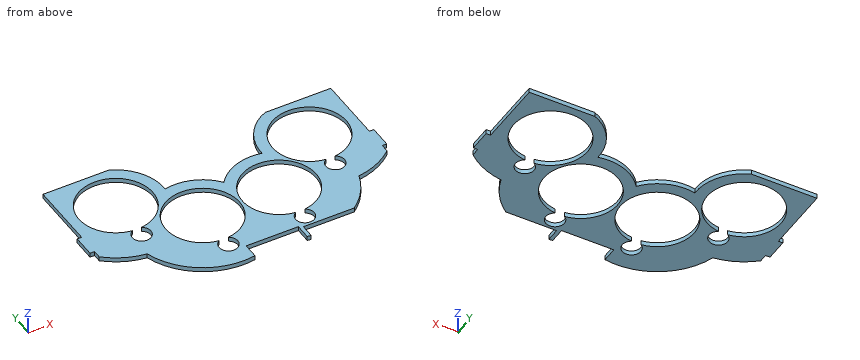
from build123d import *

# Parameters (mm, degrees)
EXTRUDE_1_DEPTH = 6


with BuildPart() as part:
    # Эскиз1 → Бобышка-Вытянуть1 (new body)
    with BuildSketch(Plane.XY):
        with BuildLine():
            Line((424, 250), (424, 160))
            Line((424, 160), (430, 160))
            Line((430, 160), (430, 130))
            Line((430, 130), (424, 130))
            Line((424, 130), (424, 118.979785419))
            ThreePointArc((424, 118.979785419), (400.249049588, 103.530628738), (372.998295097, 95.773021676))
            ThreePointArc((372.998295097, 95.773021676), (359.88843335, 69.223630945), (339.241493801, 48))
            Line((339.241493801, 48), (271, 48))
            Line((271, 48), (271, 29.720915629))
            ThreePointArc((271, 29.720915629), (268.495114821, 30.054927971), (266, 30.455447679))
            Line((266, 30.455447679), (266, 51))
            Line((266, 51), (196, 51))
            Line((196, 51), (196, 30.455447679))
            ThreePointArc((196, 30.455447679), (130.198007186, 42.960646788), (89.001704904, 95.773021676))
            ThreePointArc((89.001704904, 95.773021676), (61.750950412, 103.530628738), (38, 118.979785419))
            Line((38, 118.979785419), (38, 130))
            Line((38, 130), (32, 130))
            Line((32, 130), (32, 160))
            Line((32, 160), (38, 160))
            Line((38, 160), (38, 250))
            Line((38, 250), (126.096189432, 250))
            ThreePointArc((126.096189432, 250), (155.836604626, 225.049778093), (166.051782667, 187.59772866))
            ThreePointArc((166.051782667, 187.59772866), (201.928287817, 185.126127233), (231, 163.958510782))
            ThreePointArc((231, 163.958510782), (260.071712183, 185.126127233), (295.948217333, 187.59772866))
            ThreePointArc((295.948217333, 187.59772866), (306.163395374, 225.049778093), (335.903810568, 250))
            Line((335.903810568, 250), (424, 250))
        make_face()
        with BuildLine():
            ThreePointArc((107.24460838, 140.883333333), (101.096189432, 239.5), (94.947770485, 140.883333333))
            ThreePointArc((94.947770485, 140.883333333), (101.096189432, 117.5), (107.24460838, 140.883333333))
        make_face(mode=Mode.SUBTRACT)
        with BuildLine():
            ThreePointArc((185.845397449, 74.929440215), (179.696978501, 173.546106882), (173.548559554, 74.929440215))
            ThreePointArc((173.548559554, 74.929440215), (179.696978501, 51.546106882), (185.845397449, 74.929440215))
        make_face(mode=Mode.SUBTRACT)
        with BuildLine():
            ThreePointArc((288.451440446, 74.929440215), (282.303021499, 173.546106882), (276.154602551, 74.929440215))
            ThreePointArc((276.154602551, 74.929440215), (282.303021499, 51.546106882), (288.451440446, 74.929440215))
        make_face(mode=Mode.SUBTRACT)
        with BuildLine():
            ThreePointArc((367.052229515, 140.883333333), (360.903810568, 239.5), (354.75539162, 140.883333333))
            ThreePointArc((354.75539162, 140.883333333), (360.903810568, 117.5), (367.052229515, 140.883333333))
        make_face(mode=Mode.SUBTRACT)
    extrude(amount=EXTRUDE_1_DEPTH)


solid = part.part
Geometry: final body of the model. Coordinates: model frame, mm. Give positions to 0.01 mm unless a question says otherwise; leave off trailing zeros. Loops run counter-clockwise (first coordinate to the right, second up) from the corner with the lowest first, then second, coordinate; pieces in that order, holes last. Notation, with made-up numbers: (-35, 61) - (-6, 61) arc R20 ccw to (-6, 92) - close; hole circle Ø10 at (45.25, 86). An arc over 180 degrees is marked (long way). Answer as CSV lines item,"result". Start each with the question number.
1. Section A-A, the plane y = 178. Return loops of the section in (x, z), plus the area to 3 significant figures.
2. Ray query, L1, parallel to Y at x = 290, z = 5; L2, parallel to X at y = 211, z = 1.95; L3, parallel to X at y = 102, z = 5.7. Return the intervals inside material, ascending.
3. Section C-C, the plane x = 146.5. Return loops of the section in (y, z).
4. Pin query (flat end, axial travel): P1, Ø3, axis at y = 123.5, z = 3.5, coming from the +X side; P2, Ø3, axis at x = 36, z = 2, coming from the +Y side. Return the tip coordinate at first contact, or that it passes through.
5. Section B-B, the plane z = 3.3. Give the number of separate pieces and of enclosed holes in the cut face, plus the area to 3 significant figures.
6. Section D-D, the plane y = 100.5. Return loops of the section in (x, z), plus the area to 3 significant figures.
Answers:
1,outline,"(38, 0) - (53.07, 0) - (53.07, 6) - (38, 6) - close; (149.12, 0) - (215.95, 0) - (215.95, 6) - (149.12, 6) - close; (246.05, 0) - (312.88, 0) - (312.88, 6) - (246.05, 6) - close; (408.93, 0) - (424, 0) - (424, 6) - (408.93, 6) - close"
1,area,"983 mm2"
2,L1,"y = 48 to 54.2, 73.9 to 75.15, 172.94 to 188.59"
2,L2,"x = 38 to 56.27, 145.92 to 162.61, 299.39 to 316.08, 405.73 to 424"
2,L3,"x = 65.31 to 135.38, 224.02 to 237.98, 326.62 to 396.69"
3,outline,"(35.04, 0) - (87.33, 0) - (87.33, 6) - (35.04, 6) - close; (160.76, 0) - (170.28, 0) - (170.28, 6) - (160.76, 6) - close; (209.72, 0) - (236.51, 0) - (236.51, 6) - (209.72, 6) - close"
4,P1,"stops at x = 424"
4,P2,"stops at y = 160"
5,separate pieces,"1"
5,enclosed holes,"4"
5,area,"29,500 mm2"
6,outline,"(69.24, 0) - (136.16, 0) - (136.16, 6) - (69.24, 6) - close; (223.24, 0) - (238.76, 0) - (238.76, 6) - (223.24, 6) - close; (325.84, 0) - (392.76, 0) - (392.76, 6) - (325.84, 6) - close"
6,area,"896 mm2"
